Model file for the job. Use its own axes, mm. A direction names the side the tool comes from. Give positions to 0.01 mm unless a question says otherwise; leave off trailing zeros. Order: outer loops, then holes, each group sorted by start corner. A loop starts at its lowest first (then second) coordinate and runs counter-clockwise, first axis right, second up. Notation, with made-up numbers: (-10.75, -21) - (4.25, -21) arc R21 cw to (4.25, 0) - close; hole circle Ø1 at (1.25, 21.25). An arc over 180 degrees is marked (long way). Use CSV: the item, a comma, the result in double quotes. Start each with the question number.
(1) Band-saw the part on C-C, the plane x = 3. Give the cut face in (y, z).
(2) Band-saw the part on D-D, the plane y = 38.5. Give the cut face in (x, z) (1 decimal), then the cut area to 3 significant figures.
(3) Drop flat-ended pins along their axis: pin 1 Ø2 at (y, z) = (33, 24) entering from -X; pin 2 Ø1.5 at (y, z) = (-69, -6) entering from -X; pin 3 Ø5 at (x, y) = (7.5, -3.5) entering from +Z. Give the stop position or say it passes through.
(4) Tool access for faces 4 (the flat face through (26, -150, -16)), 5 (the flat face through (30, -130, -7)): list every direction of +Z, -Z, +X, -X, +Y, -Y with a clear straight run to the whole face (end or side of a thin tool).
(5) Band-saw the part on A-A, the plane z = 0. Give the cut face in (x, y) (1 decimal), then the cut area to 3 significant figures.
(6) Probe L1, parallel to Z at x = 0, y = 40.5 (1 decimal); L2, parallel to Z at x = -25, y = 109. List the from-to ranges inside material, lowest first.
(7) Band-saw the part on B-B, the plane x = -17.5. Give the cut face in (y, z), then the cut area to 3 significant figures.
(8) Pull direction X, two halves, no side cores. Call faces 1 (the flat face through (30, -117.8, -7)), 2 (the cylindrical face through (1.326, -2.1, -30.133)), 3 (the cylindrical face through (26.28, 2.1, 16.75)): +X half, -X half, draft (parallel to the pull), parting line (faces both ways), or undercut.
from build123d import *

# Parameters (mm, degrees)
SKETCH1_R           = 31.165
SKETCH1_R_2         = 30.1625
BOSS_EXTRUDE1_DEPTH = 150
SKETCH2_W           = 31.165
SKETCH2_H           = 62.33
SLOT_DEPTH          = 12.2


with BuildPart() as part:
    # Sketch1 → Boss-Extrude1 (new, symmetric)
    with BuildSketch(Plane(origin=(0, 0, 0), x_dir=(1, 0, 0), z_dir=(0, 1, 0))):
        with Locations(Location((0, 0, 0), (0, 0, 270))):
            Circle(SKETCH1_R)
        with Locations(Location((0, 0, 0), (0, 0, 270))):
            Circle(SKETCH1_R_2, mode=Mode.SUBTRACT)
    extrude(amount=BOSS_EXTRUDE1_DEPTH, both=True)

    # Sketch2 → Slot (cut)
    with BuildSketch(Plane(origin=(0, -130, 0), x_dir=(-1, 0, 0), z_dir=(0, -1, 0))):
        with Locations((-15.5825, 0)):
            Rectangle(SKETCH2_W, SKETCH2_H)
    extrude(amount=-SLOT_DEPTH, mode=Mode.SUBTRACT)


solid = part.part
Answer block:
1,outline,"(-150, -31.02) - (-130, -31.02) - (-130, -30.01) - (-150, -30.01) - close; (-150, 30.01) - (-130, 30.01) - (-130, 31.02) - (-150, 31.02) - close; (-117.8, -31.02) - (150, -31.02) - (150, -30.01) - (-117.8, -30.01) - close; (-117.8, 30.01) - (150, 30.01) - (150, 31.02) - (-117.8, 31.02) - close"
2,outline,"circle Ø62.3 at (0, 0); hole circle Ø60.3 at (0, 0)"
2,area,"193 mm2"
3,pin 1,"stops at x = -21.03"
3,pin 2,"stops at x = -30.72"
3,pin 3,"stops at z = 30.76"
4,face 4,"+Z, -Z, +X, -X, -Y"
4,face 5,"+Z, -Z, +X"
5,outline,"(-31.2, -150) - (-30.2, -150) - (-30.2, 150) - (-31.2, 150) - close; (30.2, -150) - (31.2, -150) - (31.2, -130) - (30.2, -130) - close; (30.2, -117.8) - (31.2, -117.8) - (31.2, 150) - (30.2, 150) - close"
5,area,"589 mm2"
6,L1,"z = -31.2 to -30.2, 30.2 to 31.2"
6,L2,"z = -18.61 to -16.88, 16.88 to 18.61"
7,outline,"(-150, -25.79) - (150, -25.79) - (150, -24.57) - (-150, -24.57) - close; (-150, 24.57) - (150, 24.57) - (150, 25.79) - (-150, 25.79) - close"
7,area,"733 mm2"
8,face 1,"draft"
8,face 2,"undercut"
8,face 3,"parting line"
